Model file for the job. Use its own axes, mm. Face numbers are marked on the shaded views. Round coordinates to 2 decimals unless told otherwise and drop trailing zeros. Loops run counter-clockwise (first coordinate to the right, second up) from the corner with the lowest first, then second, coordinate; pieces in that order, holes last.
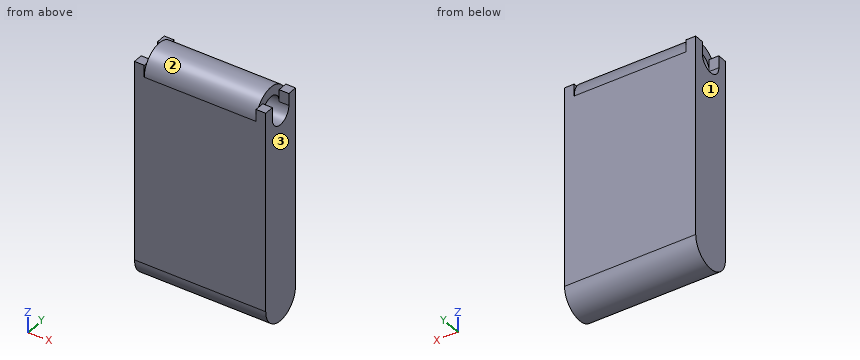
from build123d import *

# Parameters (mm, degrees)
SKETCH1_R                = 2.01676
BOSS_EXTRUDE2_DEPTH      = 10.88771
BOSS_EXTRUDE2_DEPTH_BACK = 10.88771
SKETCH2_R                = 3.62966
CUT_EXTRUDE1_DEPTH       = 1.6129
BOSS_EXTRUDE3_DEPTH      = 1.6129


with BuildPart() as part:
    # Sketch1 → Boss-Extrude2 (new body, two sides)
    with BuildSketch(Plane(origin=(0, 0, 0), x_dir=(0, 0, -1), z_dir=(1, 0, 0))) as boss_extrude2_sk:
        with BuildLine():
            Line((-15.72768, 3.62966), (15.72768, 3.62966))
            ThreePointArc((15.72768, 3.62966), (19.35734, 0), (15.72768, -3.62966))
            Line((15.72768, -3.62966), (-15.72768, -3.62966))
            ThreePointArc((-15.72768, -3.62966), (-19.35734, 0), (-15.72768, 3.62966))
        make_face()
        with Locations((-15.72768, 0)):
            Circle(SKETCH1_R, mode=Mode.SUBTRACT)
    extrude(amount=BOSS_EXTRUDE2_DEPTH)
    extrude(boss_extrude2_sk.sketch, amount=-BOSS_EXTRUDE2_DEPTH_BACK)

    # Sketch2 → Cut-Extrude1 (cut)
    with BuildSketch(Plane(origin=(10.88771, 0, 0), x_dir=(0, 0, -1), z_dir=(1, 0, 0))):
        with Locations((-15.72768, 0)):
            Circle(SKETCH2_R)
    cut_extrude1 = extrude(amount=-CUT_EXTRUDE1_DEPTH, mode=Mode.SUBTRACT)

    # Mirror1: Cut-Extrude1 across plane
    add(cut_extrude1.mirror(Plane(origin=(0, 0, 0), x_dir=(0, 0, 1), z_dir=(1, 0, 0))), mode=Mode.SUBTRACT)

    # Sketch3 → Boss-Extrude3 (add)
    with BuildSketch(Plane(origin=(10.88771, 0, 0), x_dir=(0, 0, -1), z_dir=(1, 0, 0))):
        with BuildLine():
            Line((-17.74444, -2.01676), (-17.74444, -3.62966))
            Line((-17.74444, -3.62966), (-15.72768, -3.62966))
            ThreePointArc((-15.72768, -3.62966), (-12.09802, 0), (-15.72768, 3.62966))
            Line((-15.72768, 3.62966), (-17.74444, 3.62966))
            Line((-17.74444, 3.62966), (-17.74444, 2.01676))
            Line((-17.74444, 2.01676), (-15.72768, 2.01676))
            ThreePointArc((-15.72768, 2.01676), (-13.71092, 0), (-15.72768, -2.01676))
            Line((-15.72768, -2.01676), (-17.74444, -2.01676))
        make_face()
    boss_extrude3 = extrude(amount=-BOSS_EXTRUDE3_DEPTH)

    # Mirror2: Boss-Extrude3 across plane
    add(boss_extrude3.mirror(Plane(origin=(0, 0, 0), x_dir=(0, 0, 1), z_dir=(1, 0, 0))))


solid = part.part
Q1. Flat gauge pins, fed straight in: P1, Ø1.8, axis at y = -1, z = 18, coming from the -X side; P2, Ø1.3, axis at x = 10.5, y = 3, coming from the +Z side; P3, Ø3, axis at y = -0.5, z = 18, coming from the +X side; P4, Ø3, axis at y = 0, z = 15.73, coming from the -X side. Where does each tip first touch, or does it go through?
Q2. Slice it at B-B on x = -0.75. Give the cut face in (y, z), plus the area to 3 significant figures.
Q3. Pull direction X, two halves, no side cores. Call the marked faces 1, 2 and 3: pulls with the +X half, pulls with the -X half, needs draft (parallel to the pull), parting line crosses it, or undercut.
Q4. Slice it at A-A on y = 0. Give the cut face in (x, z).
Q5. Probe line 1 (Z direction, x = 1, y = 0); line 2 (Y direction, x = -4.25, z = 14.5); line 3 (Z direction, x = 1.25, y = -1). List the from-to ranges inside material, lowest first.
Q6. Slice it at C-C on z = -17. Give the cut face in (x, y).
Reply:
1. P1: stops at x = -9.27
1. P2: stops at z = 17.74
1. P3: stops at x = 9.27
1. P4: passes through
2. outline: (-3.63, -15.73) arc R3.63 ccw to (3.63, -15.73) - (3.63, 15.73) arc R3.63 ccw to (-3.63, 15.73) - close; hole circle Ø4.03 at (0, 15.73)
2. area: 257 mm2
3. face 1: pulls with the -X half
3. face 2: undercut
3. face 3: pulls with the +X half
4. outline: (-10.89, -19.36) - (10.89, -19.36) - (10.89, 13.71) - (-10.89, 13.71) - close; (-9.27, 17.74) - (9.27, 17.74) - (9.27, 19.36) - (-9.27, 19.36) - close
5. line 1: z = -19.36 to 13.71, 17.74 to 19.36
5. line 2: y = -3.63 to -1.6, 1.6 to 3.63
5. line 3: z = -19.22 to 13.98, 17.48 to 19.22
6. outline: (-10.89, -3.4) - (10.89, -3.4) - (10.89, 3.4) - (-10.89, 3.4) - close
